```python
from build123d import *

# Parameters (mm, degrees)
SKETCH1_R           = 2
SKETCH1_R_2         = 3
SKETCH1_R_3         = 5
BOSS_EXTRUDE1_DEPTH = 6
FILLET1_R           = 20
FILLET2_R           = 10
CUT_EXTRUDE1_DEPTH  = 697.921769691
FILLET3_R           = 5
SKETCH3_R           = 2
CUT_EXTRUDE2_DEPTH  = 697.921769691
SKETCH9_R           = 2
CUT_EXTRUDE4_DEPTH  = 697.921769691


with BuildPart() as part:
    # Sketch1 → Boss-Extrude1 (new body)
    # profile 1 of 2: a face of its own
    with BuildSketch(Plane.XY):
        Polygon((0, 146.44), (0, 0), (30, 0), (30, 50), (60, 80), (96.44, 116.44), (354.44, 116.44), (418.384389798, 80), (471.027959885, 50), (582.094928321, -13.293751689), (662.443379532, -109.049307079), (685.424712826, -89.765678789), (487.224614872, 146.44), align=None)
        with Locations((668.791745302, -93.279137389)):
            Circle(SKETCH1_R, mode=Mode.SUBTRACT)
        with Locations((654.650417888, -76.42615964)):
            Circle(SKETCH1_R, mode=Mode.SUBTRACT)
        with Locations((15, 15)):
            Circle(SKETCH1_R_2, mode=Mode.SUBTRACT)
        with Locations((15, 115)):
            Circle(SKETCH1_R_2, mode=Mode.SUBTRACT)
    # profile 2 of 2: a face of its own
    with BuildSketch(Plane.XY):
        Polygon((60, 80), (30, 50), (471.027959885, 50), (418.384389798, 80), align=None)
        with Locations((240.003736421, 65)):
            Circle(SKETCH1_R_3, mode=Mode.SUBTRACT)
    extrude(amount=BOSS_EXTRUDE1_DEPTH)

    # Fillet1
    fillet1_edges = [part.edges().sort_by_distance(p)[0] for p in [
        (30, 50, 3),
    ]]
    fillet(fillet1_edges, radius=FILLET1_R)

    # Fillet2
    fillet2_edges = [part.edges().sort_by_distance(p)[0] for p in [
        (418.384389798, 80, 3),
        (354.44, 116.44, 3),
        (96.44, 116.44, 3),
        (60, 80, 3),
        (30, 0, 3),
        (0, 0, 3),
        (0, 146.44, 3),
        (487.224614872, 146.44, 3),
        (685.424712826, -89.765678789, 3),
        (662.443379532, -109.049307079, 3),
        (582.094928321, -13.293751689, 3),
        (471.027959885, 50, 3),
    ]]
    fillet(fillet2_edges, radius=FILLET2_R)

    # Sketch2 → Cut-Extrude1 (cut, through all)
    with BuildSketch(Plane.XY.offset(6)):
        Polygon((404.933023937, 116.44), (473.235385128, 116.44), (526.571079334, 52.876994817), (478.976018523, 80), (468.877413735, 80), align=None)
    extrude(amount=-CUT_EXTRUDE1_DEPTH, mode=Mode.SUBTRACT)

    # Fillet3
    fillet3_edges = [part.edges().sort_by_distance(p)[0] for p in [
        (468.877413735, 80, 3),
        (404.933023937, 116.44, 3),
        (473.235385128, 116.44, 3),
        (526.571079334, 52.876994817, 3),
        (478.976018523, 80, 3),
    ]]
    fillet(fillet3_edges, radius=FILLET3_R)

    # Sketch3 → Cut-Extrude2 (cut, through all)
    with BuildSketch(Plane.XY.offset(6)):
        with Locations((609.65528521, -22.803048622)):
            Circle(SKETCH3_R)
        with Locations((440.003736421, 65)):
            Circle(SKETCH3_R)
        with Locations((535.979779495, 65)):
            Circle(SKETCH3_R)
        with Locations((480.23, 131.44)):
            Circle(SKETCH3_R)
        with Locations((305.003736421, 65)):
            Circle(SKETCH3_R)
        with Locations((331.395769145, 131.44)):
            Circle(SKETCH3_R)
        with Locations((197.561538291, 131.44)):
            Circle(SKETCH3_R)
    extrude(amount=-CUT_EXTRUDE2_DEPTH, mode=Mode.SUBTRACT)

    # Sketch9 → Cut-Extrude4 (cut, through all)
    with BuildSketch(Plane.XY.offset(6)):
        with Locations((95, 131.44)):
            Circle(SKETCH9_R)
        with Locations((63.56, 65)):
            Circle(SKETCH9_R)
    extrude(amount=-CUT_EXTRUDE4_DEPTH, mode=Mode.SUBTRACT)


solid = part.part
```
The listing builds one solid part. Answer for the finished solid, in the listing's coordinates (mm). A direction names the side the tool comes from. Coordinates: 2 decimals unless noted, no trailing zeros. Write each loop counter-clockwise with the first axis right and the second up, starting at its lowest first coordinate (ties: lowest second). Pieces come first, ordered by that corner, then holes. Notation, with made-up numbers: (-27, 29) - (-15, 29) arc R10 ccw to (-15, 47) - close; hole circle Ø2 at (68.5, 32.5). An arc over 180 degrees is marked (long way). One line per item, written item: value.
1) Find section B-B (z = 3.5). Count the separate pieces of the cut face and the enclosed holes in it, and give its area (3 significant figures).
Geometry check:
separate pieces: 1
enclosed holes: 16
area: 46,900 mm2
2) Find section D-D (x = 632.5). Give the vertices of the cut face in (y, z), and give its area (3 significant figures).
Geometry check:
outline: (-73.36, 0) - (-26.69, 0) - (-26.69, 6) - (-73.36, 6) - close
area: 280 mm2
3) Find section C-C (y = -52.5). Give the vertices of the cut face in (x, z).
Geometry check:
outline: (614.99, 0) - (654.16, 0) - (654.16, 6) - (614.99, 6) - close
4) Each of these flat-tipped pins is pushed along its axis until it touches: pin 1 Ø4.5 at (x, y) = (197.56, 131.44) entering from -Z; pin 2 Ø10 at (x, y) = (288, 107.5) entering from -Z; pin 3 Ø3 at (x, z) = (198.5, 2) entering from -Y; pin 4 Ø3 at (y, z) = (24, 3.5) entering from +X. Where does it stop, or does it pass through?
Geometry check:
pin 1: stops at z = 0
pin 2: passes through
pin 3: stops at y = 50
pin 4: stops at x = 591.22
5) For a pull along Y with two mould halves and no side action, classify faces 4 (the flat face through (314, 77, 6)), 5 (the flat face through (444.853, 93.691, 3.042)), 6 (the flat face through (491.45, 94.73, 3.04)), 7 (the flat face through (526.18, 18.57, 2.96)) as pulls with the +Y half, pulls with the -Y half, needs draft (parallel to the pull), parting line crosses it, or undercut.
Geometry check:
face 4: needs draft
face 5: undercut
face 6: undercut
face 7: pulls with the -Y half
6) Consider line 1 along Y through (x, z) = (95, 3.55); line 2 along X through (y, z) = (131.44, 3); line 3 along X through (y, z) = (107.5, 2). Determine where each line is inside the solid, lowest interval first. Write a range as from..to.
Geometry check:
line 1: y = 50..80, 114.74..129.44, 133.44..146.44
line 2: x = 0..93, 97..195.56, 199.56..329.4, 333.4..478.23, 482.23..499.81
line 3: x = 0..87.5, 370.13..420.73, 480.74..519.9
7) A tool of negligible diameter and unlimited length cuts with its end or side. For faces 1 (the flat face through (370.964, 107.023, 2.958)), 2 (the flat face through (619.12, -57.42, 2.96)), 3 (the cylindrical face through (36.014, 44.297, 3.042)), from which of +Z, -Z, +X, -X, +Y, -Y can it reach the whole face along a straight path? Write none if from no direction.
Geometry check:
face 1: +Z, -Z
face 2: +Z, -Z, -X, -Y
face 3: +Z, -Z, -Y
8) Find section A-A (x = 160.5). Give the vertices of the cut face in (y, z).
Geometry check:
outline: (50, 0) - (80, 0) - (80, 6) - (50, 6) - close; (116.44, 0) - (146.44, 0) - (146.44, 6) - (116.44, 6) - close
